CAD build for the part. Positions are in the model's coordinates, mm. A direction names the side the tool comes from. Coordinates: 2 decimals unless noted, no trailing zeros. Write each loop counter-clockwise with the first axis right and the second up, starting at its lowest first coordinate (ties: lowest second). Pieces come first, ordered by that corner, then holes. Notation, with made-up numbers: (81, 58.25) - (88, 58.25) arc R11 cw to (88, 76.25) - close; hole circle Ø1 at (-31.5, 21.5). An arc over 180 degrees is marked (long way). Answer in a Markdown table with one row per item. Add a question column.
Q1. 3-axis set-ups, long thin cutter, end or side, ignore diameter. For faces 1 (the cylindrical face through (-11.521, 12.622, 75.897)), 2 (the flat face through (-10, 0, 45)), 3 (the flat face through (-13, 22.5, 37)): which of +Z, -Z, +X, -X, +Y, -Y reach the whole face in a straight line?
Q2. Band-saw the part on C-C (z = 9). List the corners of the cut face in (x, y), and give its area (3 significant figures).
Q3. Band-saw the part on D-D (y = -6). List the corners of the cut face in (x, z), and give its area (3 significant figures).
Q4. Drill centre lines: line 1 along Y through (x, z) = (-12.15, 73); line 2 along Z through (x, y) = (-12.25, 12.75); line 3 along X through (y, z) = (-12.5, 5.5). Where is each one in solid material? Low to high. Write a range as from..to.
Q5. Band-saw the part on A-A (z = 30.5). List the corners of the cut face in (x, y), and give its area (3 significant figures).
Q6. Pin check, flat tips, straight feed: pin 1 (3 mm diameter, centred on x = -5, y = 0, fed in from -Z); pin 2 (4.5 mm diameter, centred on y = 14, z = 31, fed in from +X); pin 3 (3.5 mm diameter, centred on y = -12.75, z = 73, fed in from +X); pin 4 (2 mm diameter, centred on x = -8, y = -2, fed in from -Z). Stop position of each tip, or through.
Q7. Two-plate mould, pull along X, no slides. Class faces 4 (the cylindrical face through (-16.5, -12.8, 32)), 5 (the cylindrical face through (4.92, 14.3, 4.93)), 6 (the flat face through (-20, 0, 39)): +X half, -X half, draft (parallel to the pull), parting line (faces both ways), or undercut.
Q8. Band-saw the part on B-B (y = 0). List the corners of the cut face in (x, z), and give its area (3 significant figures).
Autodesk Inventor part; units mm, degrees
ref_plane "YZ Plane" through (0, 0, 0) normal (1, 0, 0) x (0, 1, 0)
ref_plane "XZ Plane" through (0, 0, 0) normal (0, 1, 0) x (-1, 0, 0)
ref_plane "XY Plane" through (0, 0, 0) normal (0, 0, 1) x (1, 0, 0)
sketch "Sketch1" plane through (0, 0, 0) normal (0, 0, 1) x (1, 0, 0)
  line L0 (-10, -22.5) -> (10, -22.5)
  line L1 (10, -22.5) -> (10, 22.5)
  line L2 (10, 22.5) -> (-10, 22.5)
  line L3 (-10, 22.5) -> (-10, -22.5)
  line L4 (-10, -22.5) -> (10, 22.5) construction
  line L5 (10, -22.5) -> (-10, 22.5) construction
  line L6 (-10, 22.5) -> (-20, 22.5)
  line L7 (-20, 22.5) -> (-20, -22.5)
  line L8 (-20, -22.5) -> (-10, -22.5)
  line L9 (-10, -22.5) -> (-10, 22.5)
  point P0 (0, 0)
  dimension "d0" = 20
  dimension "d1" = 45
  dimension "d2" = 10
extrude "Extrusion1" add sketch "Sketch1" along normal blind 10 contours L3 L2 L1 L0
sketch "Sketch2" plane through (0, 0, 10) normal (0, 0, 1) x (1, 0, 0)
  line L0 (5, -12.5) -> (-5, -12.5) construction
  line L1 (-5, -12.5) -> (-5, 12.5) construction
  line L2 (-5, 12.5) -> (5, 12.5) construction
  line L3 (5, 12.5) -> (5, -12.5) construction
  line L4 (5, -12.5) -> (-5, 12.5) construction
  line L5 (-5, -12.5) -> (5, 12.5) construction
  point P0 (0, 0)
  point P1 (-5, 0)
  point P2 (5, 0)
  dimension "d5" = 10
  dimension "d6" = 25
hole "Hole1" at (-5, 12.5, 10) at (5, 12.5, 10) at (5, -12.5, 10) at (-5, -12.5, 10) at (-5, 0, 10) at (5, 0, 10) direction (0, 0, -1) diameter 3.6 end through all
sketch "Sketch3" plane through (0, 0, 0) normal (0, 0, 1) x (1, 0, 0)
  line L0 (-10, 22.5) -> (-10, -22.5)
  line L1 (-10, 22.5) -> (-20, 22.5)
  line L2 (-20, 22.5) -> (-20, -22.5)
  line L3 (-20, -22.5) -> (-10, -22.5)
  line L4 (-10, -22.5) -> (-10, 22.5)
  point P0 (0, 0)
  dimension "d14" = 10
extrude "Extrusion2" add sketch "Sketch3" along normal blind 80
sketch "Sketch4" plane through (-10, -22.5, 10) normal (1, 0, 0) x (0, 0, -1)
  line L0 (-63, 9.75) -> (-20.5, 9.75)
  line L1 (-20.5, 9.75) -> (-20.5, 35.25)
  line L2 (-20.5, 35.25) -> (-63, 35.25)
  line L3 (-63, 35.25) -> (-63, 9.75)
  line L4 (-63, 9.75) -> (-20.5, 35.25) construction
  line L5 (-20.5, 9.75) -> (-63, 35.25) construction
  line L6 (0, 0) -> (0, 45)
  line L7 (-70, 0) -> (-70, 45)
  line L8 (0, 45) -> (-70, 45)
  point P0 (10, 22.5)
  point P1 (-41.75, 22.5)
  point P2 (-70, 22.5)
  dimension "d17" = 42.5
  dimension "d18" = 25.5
  dimension "d19" = 7
hole "Hole2" at (-10, 12.75, 73) at (-10, -12.75, 73) at (-10, 12.75, 30.5) at (-10, -12.75, 30.5) direction (-1, 0, 0) diameter 3 end through all
sketch "Sketch5" plane through (-10, -22.5, 10) normal (1, 0, 0) x (0, 0, -1)
  circle A0 centre (-63, 35.25) radius 1.5
  circle A1 centre (-20.5, 35.25) radius 1.5
  circle A2 centre (-20.5, 9.75) radius 1.5
  circle A3 centre (-63, 9.75) radius 1.5
  point P0 (10, 22.5)
hole "Hole3" at (-10, 12.75, 73) at (-10, 12.75, 30.5) at (-10, -12.75, 30.5) at (-10, -12.75, 73) direction (-1, 0, 0) diameter 5.8 depth 3
fillet "Fillet1" radius 5 4 edges at (-15, 22.5, 80) (-15, -22.5, 80) (10, 22.5, 5) (10, -22.5, 5)
properties part number "Uchwyt_konwerter" material "PET Plastic"
Checked values:
| question | item | result |
|---|---|---|
| 1 | face 1 | +X |
| 1 | face 2 | +Z, +X, +Y, -Y |
| 1 | face 3 | +Z, -Z, +X, -X, +Y |
| 2 | outline | (-20, -22.5) - (5, -22.5) arc R5 ccw to (10, -17.5) - (10, 17.5) arc R5 ccw to (5, 22.5) - (-20, 22.5) - close; hole circle Ø3.6 at (-5, -12.5); hole circle Ø3.6 at (-5, 0); hole circle Ø3.6 at (-5, 12.5); hole circle Ø3.6 at (5, -12.5); hole circle Ø3.6 at (5, 0); hole circle Ø3.6 at (5, 12.5) |
| 2 | area | 1,280 mm² |
| 3 | outline | (-20, 0) - (10, 0) - (10, 10) - (-10, 10) - (-10, 80) - (-20, 80) - close |
| 3 | area | 1,000 mm² |
| 4 | line 1 | y = -22.5..-15.65, -9.85..9.85, 15.65..22.5 |
| 4 | line 2 | z = 0..27.6, 33.4..70.1, 75.9..80 |
| 4 | line 3 | x = -20..-6.8, -3.2..3.2, 6.8..10 |
| 5 | outline | (-20, -22.5) - (-10, -22.5) - (-10, -15.65) - (-13, -15.65) - (-13, -14.25) - (-20, -14.25) - close; (-20, -11.25) - (-13, -11.25) - (-13, -9.85) - (-10, -9.85) - (-10, 9.85) - (-13, 9.85) - (-13, 11.25) - (-20, 11.25) - close; (-20, 14.25) - (-13, 14.25) - (-13, 15.65) - (-10, 15.65) - (-10, 22.5) - (-20, 22.5) - close |
| 5 | area | 373 mm² |
| 6 | pin 1 | passes through |
| 6 | pin 2 | stops at x = -10 |
| 6 | pin 3 | stops at x = -13 |
| 6 | pin 4 | stops at z = 0 |
| 7 | face 4 | draft |
| 7 | face 5 | undercut |
| 7 | face 6 | -X half |
| 8 | outline | (-20, 0) - (-6.8, 0) - (-6.8, 10) - (-10, 10) - (-10, 80) - (-20, 80) - close; (-3.2, 0) - (3.2, 0) - (3.2, 10) - (-3.2, 10) - close; (6.8, 0) - (10, 0) - (10, 10) - (6.8, 10) - close |
| 8 | area | 928 mm² |
